Here's how the part is built. I have some questions about the finished solid (model axes, mm). Face numbers are marked on the shaded views. A direction names the side the tool comes from. Round coordinates to 2 decimals unless told otherwise and drop trailing zeros. Order: outer loops, then holes, each group sorted by start corner. A loop starts at its lowest first (then second) coordinate and runs counter-clockwise, first axis right, second up. Notation, with made-up numbers: M -34.75,0 L -10.75,0 A14 cw -10.75,10 Z; hole C 40,-12.5 d11. An arc over 180 degrees is marked long. Write each question's results on one line, items separated by ' | '. Start each with the question number.
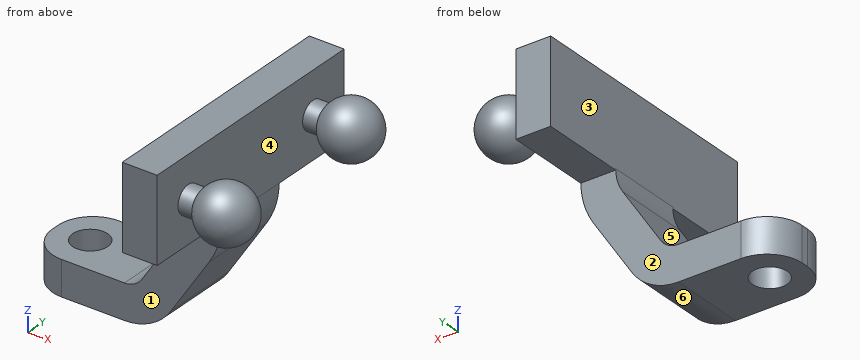
```python
from build123d import *

# Parameters (mm, degrees)
EXTRUDE_1_DEPTH     = 2.75
SKETCH_2_R          = 1.25
CUT_EXTRUDE_1_DEPTH = 10
FILLET_2_R          = 2.5
EXTRUDE_2_REACH     = 21.1
SKETCH_4_W          = 6
SKETCH_4_H          = 18
SKETCH_5_R          = 1
EXTRUDE_3_DEPTH     = 1


with BuildPart() as part:
    # 草图1 → 凸台-拉伸1 (new, symmetric)
    with BuildSketch(Plane(origin=(0, 0, 0), x_dir=(1, 0, 0), z_dir=(0, 1, 0))):
        with BuildLine():
            Line((0, 0), (7, 0))
            ThreePointArc((7, 0), (8.907645559, -0.484194485), (10.353455389, -1.819555789))
            Line((10.353455389, -1.819555789), (13.08620622, -6.022441585))
            ThreePointArc((13.08620622, -6.022441585), (13.76673936, -7.496994372), (14, -9.104172255))
            Line((14, -9.104172255), (14, -15))
            Line((14, -15), (11.5, -15))
            Line((11.5, -15), (11.5, -9.104172255))
            ThreePointArc((11.5, -9.104172255), (11.369889965, -8.207707378), (10.990296602, -7.385219216))
            Line((10.990296602, -7.385219216), (8.257545771, -3.182333421))
            ThreePointArc((8.257545771, -3.182333421), (7.715367085, -2.681572932), (7, -2.5))
            Line((7, -2.5), (0, -2.5))
            Line((0, -2.5), (0, 0))
        make_face()
    extrude(amount=EXTRUDE_1_DEPTH, both=True)

    # 草图2 → 切除-拉伸1 (cut)
    with BuildSketch(Plane(origin=(0, 0, 0), x_dir=(-1, 0, 0), z_dir=(0, 0, -1))):
        with Locations((-2.5, 0)):
            Circle(SKETCH_2_R)
    extrude(amount=-CUT_EXTRUDE_1_DEPTH, mode=Mode.SUBTRACT)

    # 圆角2
    fillet_2_edges = [part.edges().sort_by_distance(p)[0] for p in [
        (0, -2.75, 1.25),
        (0, 2.75, 1.25),
    ]]
    fillet(fillet_2_edges, radius=FILLET_2_R)

    # 凸台-拉伸2: up to this face of the body (flat: up to its plane)
    extrude_2_end = Plane(part.part.faces().sort_by_distance((14, 0, 12.052086128))[0])
    # 草图4 → 凸台-拉伸2 (add, up to the picked face)
    with BuildSketch(Plane.ZY.offset(-11.5), mode=Mode.PRIVATE) as extrude_2_sk1:
        with Locations((12, 0)):
            Rectangle(SKETCH_4_W, SKETCH_4_H)
    extrude_2_tool1 = split(extrude(extrude_2_sk1.sketch, amount=-EXTRUDE_2_REACH, mode=Mode.PRIVATE), bisect_by=extrude_2_end, keep=Keep.BOTH, mode=Mode.PRIVATE)
    add(extrude_2_tool1.solids().sort_by(Axis((11.5, 0, 12), (1, 0, 0)))[0])

    # 草图5 → 凸台-拉伸3 (add)
    with BuildSketch(Plane(origin=(14, 0, 0), x_dir=(0, 0, -1), z_dir=(1, 0, 0))):
        with Locations(Location((-12, 6, 0), (0, 0, 180))):
            Circle(SKETCH_5_R)
    extrude_3 = extrude(amount=EXTRUDE_3_DEPTH)

    # 草图6 → 旋转1 (revolve)
    with BuildSketch(Plane(origin=(0, 0, 12), x_dir=(-1, 0, 0), z_dir=(0, 0, -1))):
        with BuildLine():
            Line((-15, 6), (-18.732050808, 6))
            ThreePointArc((-18.732050808, 6), (-17.249688898, 7.931851653), (-15, 7))
            Line((-15, 7), (-15, 6))
        make_face()
    revolve_1 = revolve(axis=Axis((15, 6, 12), (1, 0, 0)))

    # 镜向1: 凸台-拉伸3, 旋转1 across plane
    add(extrude_3.mirror(Plane.ZX))
    add(revolve_1.mirror(Plane.ZX))


solid = part.part
```
(1) I'm going to push flat-ended pins straight in: pin 1 Ø1.8 at (y, z) = (2, 12.5) entering from -X; pin 2 Ø4.5 at (x, z) = (6.5, 4) entering from +Y; pin 3 Ø7.5 at (x, z) = (8, 4.5) entering from -Y; pin 4 Ø1 at (y, z) = (-4.5, 7) entering from +X. Where does each tip first touch, or does it pass through?
(2) I want a section at D-D on x = 15.5. Write out the boundary of the cut face in (y, z).
(3) Please list where these lines run through material, in increasing order: line 1 (Z direction, x = 12.5, y = 4.75); line 2 (Z direction, x = 5.25, y = -0.75); line 3 (Y direction, x = 2.5, z = 0.9).
(4) On a 3-axis mill with a long thin cutter (end or side, diameter ignored), from which of +Z, -Z, +X, -X, +Y, -Y can I reach the whole of each face in a straight line? I mean the marked faces 1, 2 and 3. Say none if no direction works.
(5) I want a section at B-B on z = 12. Write out the boundary of the cut face in (x, y), and give its area (3 significant figures).
(6) I want a section at C-C on y = 6. Write out the boundary of the cut face in (x, z).
(7) If we mould it in two halves opening along X, with no side actions, what happens to the marked faces 4, 5 and 6? For each: pulls with the +X half, pulls with the -X half, needs draft (parallel to the pull), parting line crosses it, or undercut.
Solutions:
1) pin 1: x = 11.5 | pin 2: y = 2.75 | pin 3: y = -2.75 | pin 4: through
2) outline: C -6,12 d3.15; C 6,12 d3.15
3) line 1: 9 to 15 | line 2: 0 to 2.5 | line 3: -2.75 to -1.25, 1.25 to 2.75
4) face 1: -Z, +X, -X, -Y | face 2: -Z, +X, -X, +Y | face 3: +Z, -X, +Y, -Y
5) outline: M 11.5,-9 L 14,-9 L 14,-7 L 15,-7 A2 ccw long 15,-5 L 14,-5 L 14,5 L 15,5 A2 ccw long 15,7 L 14,7 L 14,9 L 11.5,9 Z | area: 73.4 mm^2
6) outline: M 11.5,9 L 14,9 L 14,11 L 15,11 A2 ccw long 15,13 L 14,13 L 14,15 L 11.5,15 Z
7) face 4: undercut | face 5: pulls with the -X half | face 6: pulls with the +X half
